Can you work these out from the model? Positions are in its coordinate system, mm. A direction names the side the tool comes from. Give positions to 0.01 mm unless a question says otherwise; leave off trailing zeros. Order: outer loops, then holes, each group sorted by start corner. A loop starts at its lowest first (then second) coordinate and runs counter-clockwise, first axis right, second up. Notation, with made-up numbers: (76.5, -8) - (81.5, -8) arc R22 cw to (81.5, 16) - close; hole circle Ø1 at (-18.75, 58). An arc over 180 degrees is marked (long way). Use one line per item in the form item = value. Start each with the question number.
1) We'd pull the mould along Y, two halves only. Please class faces 1 (the cylindrical face through (0.03, 10.58, -11.22)), 2 (the cylindrical face through (-0.031, -2.681, -6.466)), 3 (the cylindrical face through (0, -11.2, 8.4)), 4 (the flat face through (2.25, -7, -97)): released by +Y, released by -Y, zero draft, split by the parting line, or undercut.
2) For pin 1 (2.5 mm diameter, centred on y = -27.68, z = -142.82, fed in from -X); pin 2 (5 mm diameter, centred on x = 1, z = -43.5, fed in from -Y); pin 3 (5 mm diameter, centred on x = -0.5, z = -69.5, fed in from +Y); pin 4 (1.3 mm diameter, centred on x = 1, z = -6.5, fed in from -Y), each with a flat end and sliding along its axis, tell me the tip position at first contact or that it passes through.
3) Which directions (+Z, -Z, +X, -X, +Y, -Y) give clear straight access to the entire face, cutting with the end or side of a thin tool? Please do faces 5 (the flat face through (-8, -73, -190)), 6 (the flat face through (0, -12, -13.224)), 7 (the flat face through (0, 14, 9)), 8 (the flat face through (0, 10, -64)), 9 (the flat face through (0, -14, -7)).
4) Please list where these lines run through material, in increasing order: probe 1 along Y at (x, z) = (-0.7, 0); probe 2 along X at (y, z) = (-59, -164); probe 3 along Y at (x, z) = (0.9, -121.61).
5) Suppose I cut it at B-B, the plane x = -14.5. Write out the boundary of the cut face in (y, z), and give its area (3 significant figures).
6) Suppose I cut it at A-A, the plane z = -187. Write out the boundary of the cut face in (x, y), and give its area (3 significant figures).
7) Suppose I cut it at C-C, the plane y = -36. Write out the boundary of the cut face in (x, z).
```python
from build123d import *

# Parameters (mm, degrees)
SKETCH_1_R          = 1.5
SKETCH_1_R_2        = 7
EXTRUDE_1_DEPTH     = 2.25
SKETCH_3_W          = 19.5
SKETCH_3_H          = 40
EXTRUDE_2_DEPTH     = 3
SKETCH_4_R          = 1.5
CUT_EXTRUDE_1_DEPTH = 227.967348396


with BuildPart() as part:
    # 草图1 → 凸台-拉伸1 (new, symmetric)
    with BuildSketch(Plane(origin=(0, 0, 0), x_dir=(0, 0, -1), z_dir=(1, 0, 0))):
        with BuildLine():
            ThreePointArc((102.736907967, -10), (110.379173808, -11.526455333), (116.85785315, -15.85785315))
            Line((116.85785315, -15.85785315), (171, -70))
            Line((171, -70), (199.284271247, -70))
            Line((199.284271247, -70), (125.142135624, 4.142135624))
            ThreePointArc((125.142135624, 4.142135624), (118.653668647, 8.47759065), (111, 10))
            Line((111, 10), (16, 10))
            ThreePointArc((16, 10), (11.149287499, 10.597149997), (6.588235294, 12.352941176))
            ThreePointArc((6.588235294, 12.352941176), (3.395498751, 13.581995002), (0, 14))
            Line((0, 14), (-18, 14))
            Line((-18, 14), (-18, 11))
            Line((-18, 11), (-13.388941598, -4.090995342))
            ThreePointArc((-13.388941598, -4.090995342), (-8.328447191, -11.253309175), (0, -14))
            Line((0, -14), (13.224243357, -14))
            Line((13.224243357, -14), (13.224243357, -10.193557234))
            ThreePointArc((13.224243357, -10.193557234), (14.608751519, -10.048447989), (16, -10))
            Line((16, -10), (102.736907967, -10))
        make_face()
        with Locations((164.036406871, -48.894271247)):
            Circle(SKETCH_1_R, mode=Mode.SUBTRACT)
        with Locations((142.823203436, -27.681067812)):
            Circle(SKETCH_1_R, mode=Mode.SUBTRACT)
        with Locations((0, -10.5)):
            Circle(SKETCH_1_R, mode=Mode.SUBTRACT)
        with Locations((-10.5, 0)):
            Circle(SKETCH_1_R, mode=Mode.SUBTRACT)
        Circle(SKETCH_1_R_2, mode=Mode.SUBTRACT)
        with Locations((10.5, 0)):
            Circle(SKETCH_1_R, mode=Mode.SUBTRACT)
        with Locations((0, 10.5)):
            Circle(SKETCH_1_R, mode=Mode.SUBTRACT)
        with Locations((40.5, 0)):
            Circle(SKETCH_1_R, mode=Mode.SUBTRACT)
        with Locations((70.5, 0)):
            Circle(SKETCH_1_R, mode=Mode.SUBTRACT)
        with Locations((121.61, -6.467864376)):
            Circle(SKETCH_1_R, mode=Mode.SUBTRACT)
        with Locations((100.5, 0)):
            Circle(SKETCH_1_R, mode=Mode.SUBTRACT)
    extrude(amount=EXTRUDE_1_DEPTH, both=True)

    # 草图3 → 凸台-拉伸2 (add)
    with BuildSketch(Plane.XZ.offset(70)):
        with Locations((-7.5, -190.144271247)):
            Rectangle(SKETCH_3_W, SKETCH_3_H)
    extrude(amount=EXTRUDE_2_DEPTH)

    # 草图4 → 切除-拉伸1 (cut, through all)
    with BuildSketch(Plane(origin=(0, -70, 0), x_dir=(1, 0, 0), z_dir=(0, 1, 0))):
        with Locations(Location((-10.25, 203.144271247, 0), (0, 0, 270))):
            Circle(SKETCH_4_R)
        with Locations(Location((-10.25, 177.144271247, 0), (0, 0, 90))):
            Circle(SKETCH_4_R)
    extrude(amount=-CUT_EXTRUDE_1_DEPTH, mode=Mode.SUBTRACT)


solid = part.part
```
Result sheet:
q1.face_1 = released by +Y
q1.face_2 = undercut
q1.face_3 = released by -Y
q1.face_4 = zero draft
q2.pin_1 = through
q2.pin_2 = -10
q2.pin_3 = 10
q2.pin_4 = -14
q3.face_5 = +Z, -Z, +X, -X, -Y
q3.face_6 = +X, -X, -Y
q3.face_7 = +Z, -Z, +X, -X, +Y
q3.face_8 = -Z, +X, -X, +Y
q3.face_9 = +Z, +X, -X, -Y
q4.probe_1 = -14 to -12, -9 to -7, 7 to 9, 12 to 14
q4.probe_2 = -2.25 to 2.25
q4.probe_3 = -20.61 to -7.97, -4.97 to 6.95
q5.outline = (-73, -210.14) - (-70, -210.14) - (-70, -170.14) - (-73, -170.14) - close
q5.area = 120 mm²
q6.outline = (-17.25, -73) - (2.25, -73) - (2.25, -57.72) - (-2.25, -57.72) - (-2.25, -70) - (-17.25, -70) - close
q6.area = 114 mm²
q7.outline = (-2.25, -165.28) - (2.25, -165.28) - (2.25, -137) - (-2.25, -137) - close
